from build123d import *

# Parameters (mm, degrees)
SKETCH_1_R          = 57.15
EXTRUDE_1_DEPTH     = 6.35
SKETCH_2_R          = 1.651
CUT_EXTRUDE_1_DEPTH = 82.071372876


with BuildPart() as part:
    # 草图1 → 凸台-拉伸1 (new body)
    with BuildSketch(Plane.XY):
        Circle(SKETCH_1_R)
    extrude(amount=EXTRUDE_1_DEPTH)

    # 草图2 → 切除-拉伸1 (cut, through all)
    with BuildSketch(Plane(origin=(0, 0, 0), x_dir=(-1, 0, 0), z_dir=(0, 0, -1))):
        with Locations((-46.743721169, 26.9875)):
            Circle(SKETCH_2_R)
        with Locations((0, 53.975)):
            Circle(SKETCH_2_R)
        with Locations((46.743721169, 26.9875)):
            Circle(SKETCH_2_R)
        with Locations((46.743721169, -26.9875)):
            Circle(SKETCH_2_R)
        with Locations((0, -53.975)):
            Circle(SKETCH_2_R)
        with Locations((-46.743721169, -26.9875)):
            Circle(SKETCH_2_R)
    extrude(amount=-CUT_EXTRUDE_1_DEPTH, mode=Mode.SUBTRACT)


solid = part.part
Work out the finished part from the listing and answer in its coordinate system (mm). Coordinates: 2 decimals unless noted, no trailing zeros. Loops run counter-clockwise (first coordinate to the right, second up) from the corner with the lowest first, then second, coordinate; pieces in that order, holes last. Notation, with made-up numbers: (69.25, -9.75) -> (97.25, -9.75) arc R23 ccw to (97.25, 12.25) -> close; hole circle Ø4 at (76, 56). An arc over 180 degrees is marked (long way). Write each question's results on one line, items separated by ' | '. Start each with the question number.
1) Find section A-A on x = 0. Determine the outline of the cut face in (y, z).
2) Find section D-D on y = 10. Determine the outline of the cut face in (x, z), then the cut area to 3 significant figures.
3) Find section B-B on z = 1.5. Count the separate pieces of the cut face and the enclosed holes in it, then the cut area to 3 significant figures.
4) Flat-ended cylindrical pins translate along their axes: P1, Ø1, axis at y = -13, z = 3, coming from the +X side; P2, Ø4, axis at x = -46.74, y = 26.99, coming from the +Z side; P3, Ø3, axis at x = -2.5, z = 3.5, coming from the -Y side; P4, Ø2, axis at x = 29.5, z = 0.5, coming from the +Y side. Find the tip coordinate at first contact, or state that the pin passes through.
5) Find section C-C on x = 33. Determine the outline of the cut face in (y, z).
6) Consider line 1 along Y through (x, z) = (0, 1.75); line 2 along Y through (x, z) = (-48, 5.75); line 3 along X through (y, z) = (52.5, 2.75). Determine where each line is inside the solid, lowest interval first.
7) The mould has two halves that part along Y. Classify faces 1 (the cylindrical face through (0.215, -52.338, 3.131)), 2 (the flat face through (-1, 1, 6.35)), 3 (the cylindrical face through (-57.095, 2.513, 3.131)): pulls with the +Y half, pulls with the -Y half, needs draft (parallel to the pull), parting line crosses it, or undercut.
Response values:
1) outline: (-57.15, 0) -> (-55.63, 0) -> (-55.63, 6.35) -> (-57.15, 6.35) -> close; (-52.32, 0) -> (52.32, 0) -> (52.32, 6.35) -> (-52.32, 6.35) -> close; (55.63, 0) -> (57.15, 0) -> (57.15, 6.35) -> (55.63, 6.35) -> close
2) outline: (-56.27, 0) -> (56.27, 0) -> (56.27, 6.35) -> (-56.27, 6.35) -> close | area: 715 mm^2
3) separate pieces: 1 | enclosed holes: 6 | area: 10,200 mm^2
4) P1: stops at x = 55.77 | P2: stops at z = 6.35 | P3: stops at y = -57.14 | P4: stops at y = 49.54
5) outline: (-46.66, 0) -> (46.66, 0) -> (46.66, 6.35) -> (-46.66, 6.35) -> close
6) line 1: y = -57.15 to -55.63, -52.32 to 52.32, 55.63 to 57.15 | line 2: y = -31.02 to -28.06, -25.92 to 25.92, 28.06 to 31.02 | line 3: x = -22.58 to -0.74, 0.74 to 22.58
7) face 1: undercut | face 2: needs draft | face 3: parting line crosses it
